Drawing for the job (mm, zero at the part's lowest x, y, z). A direction names the side the tool comes from. Coordinates: 2 decimals unless noted, no trailing zeros. Order: outer loops, then holes, each group sorted by start corner. A loop starts at its lowest first (then second) coordinate and runs counter-clockwise, first axis right, second up.
1) Cut at D-D (x = 23.5). List the corners of the cut face in (y, z).
2) Pin check, flat tips, straight feed: pin 1 Ø10 at (x, y) = (12.5, 23.5) entering from +Z; pin 2 Ø12 at (x, z) = (17.5, 14) entering from +Y. Stop position of each tip, or through.
3) Cut at C-C (z = 14). List the corners of the cut face in (x, y) (1 decimal), and give its area (3 significant figures).
4) Wall check: L1, parallel to X at y = 35, z = 14.25 (1 decimal); L2, parallel to Y at x = 32.5, z = 7.75 (1 decimal); L3, parallel to Y at x = 4, z = 4.25 (1 decimal). Give the ranges that are in metal, low to high.
5) Cut at A-A (x = 5.5). List the corners of the cut face in (y, z) (1 decimal).
6) Tool access for the marked faces 5 and 6: list every direction of +Z, -Z, +X, -X, +Y, -Y with a clear straight run to the whole face (end or side of a thin tool).
7) Mould opens along X. For the marked faces 1, 2, 3 and 4 say: +X half, -X half, draft (parallel to the pull), parting line (faces both ways), or undercut.
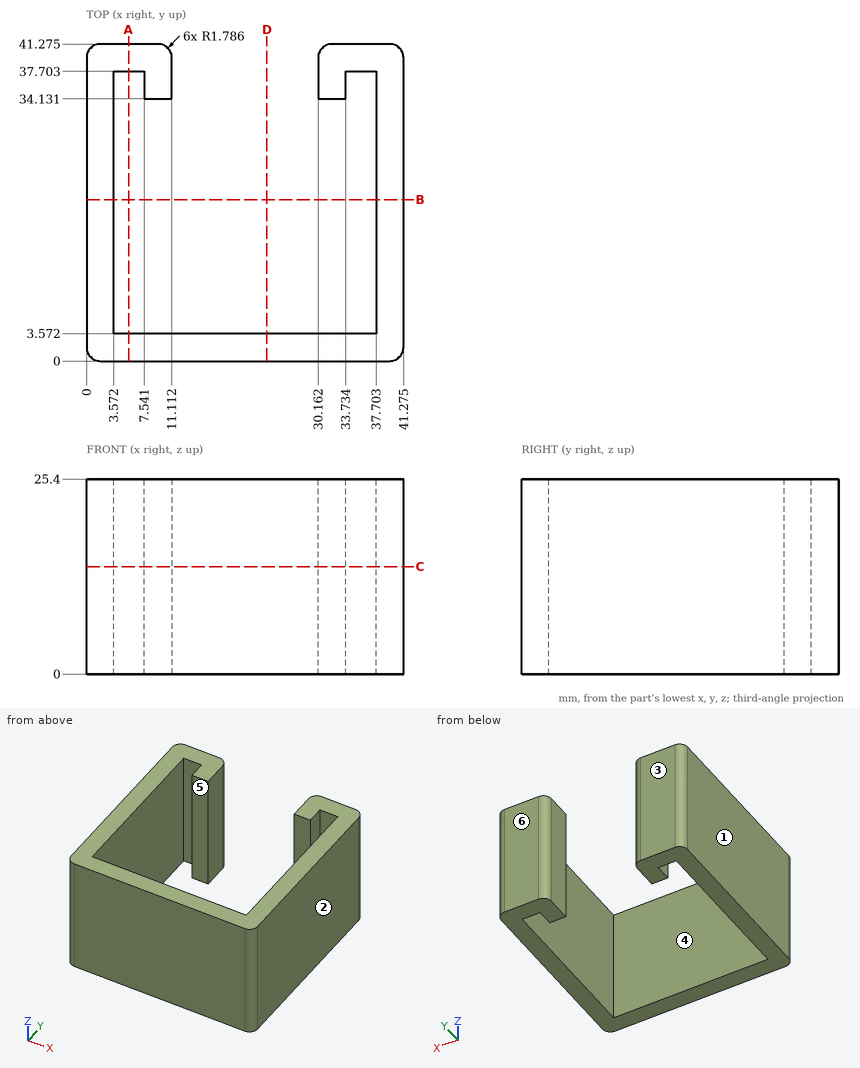
Geometry check:
1. outline: (0, 0) - (3.57, 0) - (3.57, 25.4) - (0, 25.4) - close
2. pin 1: passes through
2. pin 2: stops at y = 3.57
3. outline: (0, 1.8) arc R1.8 ccw to (1.8, 0) - (39.5, 0) arc R1.8 ccw to (41.3, 1.8) - (41.3, 39.5) arc R1.8 ccw to (39.5, 41.3) - (31.9, 41.3) arc R1.8 ccw to (30.2, 39.5) - (30.2, 34.1) - (33.7, 34.1) - (33.7, 37.7) - (37.7, 37.7) - (37.7, 3.6) - (3.6, 3.6) - (3.6, 37.7) - (7.5, 37.7) - (7.5, 34.1) - (11.1, 34.1) - (11.1, 39.5) arc R1.8 ccw to (9.3, 41.3) - (1.8, 41.3) arc R1.8 ccw to (0, 39.5) - close
3. area: 492 mm2
4. L1: x = 0 to 3.6, 7.5 to 11.1, 30.2 to 33.7, 37.7 to 41.3
4. L2: y = 0 to 3.6, 34.1 to 41.3
4. L3: y = 0 to 3.6, 37.7 to 41.3
5. outline: (0, 0) - (3.6, 0) - (3.6, 25.4) - (0, 25.4) - close; (37.7, 0) - (41.3, 0) - (41.3, 25.4) - (37.7, 25.4) - close
6. face 5: +Z, -Z
6. face 6: +Z, -Z, +X, -X, +Y
7. face 1: -X half
7. face 2: +X half
7. face 3: draft
7. face 4: undercut
